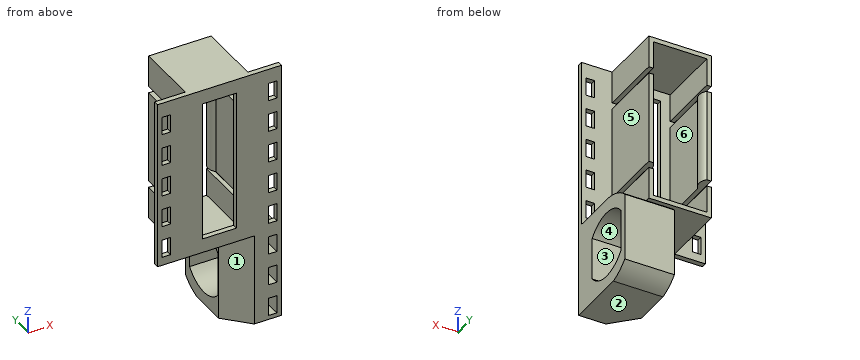
Autodesk Inventor part; units mm, degrees
ref_plane "YZ Plane" through (0, 0, 0) normal (1, 0, 0) x (0, 1, 0)
ref_plane "XZ Plane" through (0, 0, 0) normal (0, 1, 0) x (-1, 0, 0)
ref_plane "XY Plane" through (0, 0, 0) normal (0, 0, 1) x (1, 0, 0)
sketch "Sketch1" plane through (0, 0, 0) normal (0, 1, 0) x (-1, 0, 0)
  line L0 (-19.2, 26.4) -> (19.2, 26.4)
  line L1 (19.2, 26.4) -> (19.2, -26.4)
  line L2 (10.8, -26.4) -> (-10.8, -26.4)
  line L3 (-19.2, -26.4) -> (-19.2, 26.4)
  line L4 (-19.2, 26.4) -> (19.2, -26.4) construction
  line L5 (19.2, 26.4) -> (-19.2, -26.4) construction
  line L6 (-5.3, 22) -> (5.3, 22)
  line L7 (5.3, 22) -> (5.3, -22)
  line L8 (5.3, -22) -> (-5.3, -22)
  line L9 (-5.3, -22) -> (-5.3, 22)
  line L10 (-5.3, 22) -> (5.3, -22) construction
  line L11 (5.3, 22) -> (-5.3, -22) construction
  line L12 (-10.8, -26.4) -> (-10.8, -55.1)
  line L13 (-10.8, -55.1) -> (-19.2, -55.1)
  line L14 (-19.2, -55.1) -> (-19.2, -26.4)
  line L15 (10.8, -26.4) -> (19.2, -26.4)
  point P0 (0, 0)
  point P1 (13.2741, -55.1)
  dimension "d4" = 10.6
  dimension "d5" = 44
  dimension "d37" = 8.4
extrude "Extrusion1" add sketch "Sketch1" along normal blind 1.6
sketch "Sketch3" plane through (0, 1.6, 0) normal (0, 1, 0) x (1, 0, 0)
  line L0 (-5.3, 22) -> (5.3, 22)
  line L1 (5.3, -22) -> (-5.3, -22)
  line L2 (-19.2, -26.4) -> (19.2, -26.4)
  line L3 (10.8, 26.4) -> (-19.2, 26.4)
  line L4 (9.7, -26.4) -> (-9.7, -26.4)
  line L5 (-9.7, -26.4) -> (-9.7, 26.4)
  line L6 (-9.7, 26.4) -> (9.7, 26.4)
  line L7 (9.7, 26.4) -> (9.7, -26.4)
  line L8 (9.7, -26.4) -> (-9.7, 26.4) construction
  line L9 (-9.7, -26.4) -> (9.7, 26.4) construction
  line L10 (8.3, -25) -> (-8.3, -25)
  line L11 (-8.3, -25) -> (-8.3, 25)
  line L12 (-8.3, 25) -> (8.3, 25)
  line L13 (8.3, 25) -> (8.3, -25)
  line L14 (8.3, -25) -> (-8.3, 25) construction
  line L15 (-8.3, -25) -> (8.3, 25) construction
  line L16 (-9.7, 16.4) -> (-8.3, 16.4)
  line L17 (-9.7, 14.4) -> (-8.3, 14.4)
  line L18 (-9.7, -14.4) -> (-8.3, -14.4)
  line L19 (-9.7, -16.4) -> (-8.3, -16.4)
  line L20 (0, 22) -> (0, -22)
  line L21 (9.7, 16.4) -> (8.3, 16.4)
  line L22 (9.7, 14.4) -> (8.3, 14.4)
  line L23 (9.7, -14.4) -> (8.3, -14.4)
  line L24 (9.7, -16.4) -> (8.3, -16.4)
  line L25 (8.3, 16.4) -> (8.3, 14.4)
  line L26 (9.7, 16.4) -> (9.7, 14.4)
  line L27 (9.7, -14.4) -> (9.7, -16.4)
  line L28 (8.3, -14.4) -> (8.3, -16.4)
  point P0 (19.2, 26.4)
  point P1 (-10.8, 26.4)
  point P2 (0, 0)
  point P3 (0, 0)
  dimension "d8" = 19.4
  dimension "d9" = 1.4
  dimension "d10" = 1.4
  dimension "d11" = 2
  dimension "d12" = 10
  dimension "d13" = 2
  dimension "d14" = 10
extrude "Extrusion2" add sketch "Sketch3" along normal blind 20 contours L5 L19 L11 L10 L13 L24 L7 L2 | L5 L17 L11 L18 | L23 L13 L22 L7 | L5 L3 L7 L21 L13 L12 L11 L16
sketch "Sketch8" plane through (0, 1.6, 0) normal (0, 1, 0) x (1, 0, 0)
  line L0 (19.2, -26.4) -> (19.2, 55.1)
  line L1 (10.8, 55.1) -> (19.2, 55.1)
  line L2 (19.2, 55.1) -> (19.2, 26.4)
  line L3 (19.2, 26.4) -> (10.8, 26.4)
  line L4 (10.8, 26.4) -> (10.8, 55.1)
  point P0 (0, 0)
extrude "Extrusion6" add sketch "Sketch8" along normal blind 23.6
sketch "Sketch9" plane through (10.8, 0, -55.1) normal (-1, 0, 0) x (0, 0, 1)
  line L0 (28.7, 0) -> (0, 0)
  line L1 (28.7, 0) -> (28.7, 1.6)
  line L2 (28.7, 1.6) -> (28.7, 25.2)
  line L3 (0, 25.2) -> (28.7, 25.2)
  line L4 (0, 0) -> (0, 25.2)
  point P0 (55.1, 0)
extrude "Extrusion7" add sketch "Sketch9" along normal blind 7
sketch "Sketch10" plane through (19.2, 0, -55.1) normal (0, 0, -1) x (-1, 0, 0)
  line L0 (15.4, 0) -> (0, 0)
  line L1 (15.4, 25.2) -> (15.4, 0)
  line L2 (8.4, 0) -> (15.4, 7.2)
  point P0 (19.2, 0)
  dimension "d42" = 7.2
  dimension "d43" = 7
extrude "Extrusion8" cut sketch "Sketch10" against normal up to surface (28.7 mm away)
sketch "Sketch11" plane through (19.2, 0, 26.4) normal (1, 0, 0) x (0, 0, -1)
  line L0 (81.5, 0) -> (0, 0)
  line L1 (81.5, 0) -> (81.5, 25.2)
  line L2 (52.8, 25.2) -> (81.5, 25.2)
  line L3 (52.8, 1.6) -> (52.8, 25.2)
  line L4 (52.8, 7.4) -> (81.5, 7.4)
  line L5 (55.0793, 23) -> (79.6991, 23)
  arc A0 (60.8, 23) -> (60.8, 7.4) centre (67.0851, 15.2) ccw
  arc A1 (74, 7.4) -> (74, 23) centre (67.6284, 15.2) ccw
  arc A2 (56.8391, 25.2) -> (52.8, 16.1566) centre (67.0851, 15.2) ccw
  line L6 (52.8, 14.2434) -> (52.8, 7.4)
  line L7 (52.8, 7.4) -> (60.8, 7.4)
  line L8 (74.3931, 7.4) -> (81.5, 7.4)
  arc A3 (81.5, 18.9579) -> (77.9504, 25.2) centre (67.6284, 15.2) ccw
  line L9 (81.5, 11.4421) -> (81.5, 7.4)
  line L10 (77.9504, 25.2) -> (56.8391, 25.2)
  arc A4 (56.8391, 25.2) -> (52.8, 16.1566) centre (67.0851, 15.2) ccw
  line L11 (56.8391, 25.2) -> (52.8, 25.2)
  line L12 (52.8, 25.2) -> (52.8, 14.2434)
  line L13 (77.9504, 25.2) -> (81.5, 25.2)
  line L14 (81.5, 25.2) -> (81.5, 18.9579)
  arc A5 (56.8391, 25.2) -> (52.8, 16.1566) centre (67.0851, 15.2) ccw
  line L15 (52.8, 16.1566) -> (52.8, 25.2)
  line L16 (52.8, 25.2) -> (56.8391, 25.2)
  point P0 (26.4, 0)
  point P1 (77.7, 15.2)
  point P2 (57.1, 15.2)
  dimension "d46" = 7.4
  dimension "d47" = 2.2
  dimension "d48" = 8
  dimension "d49" = 13.2
  dimension "d50" = 7.8
  dimension "d51" = 3.7
  dimension "d52" = 8
  dimension "d53" = 13.2
  dimension "d54" = 7.8
  dimension "d55" = 3.7
  dimension "d56" = 4.3
  dimension "d57" = 4.3
extrude "Extrusion9" cut sketch "Sketch11" against normal up to surface (15.4 mm away) contours A3 L2 L1 | L4 A0 L5 A1 | A2 L3 L2
sketch "Sketch12" plane through (0, 0, 0) normal (0, -1, 0) x (1, 0, 0)
  line L0 (19.2, -55.1) -> (19.2, 26.4)
  line L1 (19.2, 26.4) -> (-19.2, 26.4)
  line L2 (-5.3, 22) -> (5.3, 22)
  line L3 (5.3, -22) -> (-5.3, -22)
  line L4 (15.2, 21.8) -> (17.8, 21.8)
  line L5 (17.8, 21.8) -> (17.8, 16.2)
  line L6 (17.8, 16.2) -> (15.2, 16.2)
  line L7 (15.2, 16.2) -> (15.2, 21.8)
  line L8 (0, 22) -> (0, -22)
  line L9 (15.2, 11.8) -> (17.8, 11.8)
  line L10 (17.8, 11.8) -> (17.8, 6.2)
  line L11 (17.8, 6.2) -> (15.2, 6.2)
  line L12 (15.2, 6.2) -> (15.2, 11.8)
  line L13 (15.2, 1.8) -> (17.8, 1.8)
  line L14 (17.8, 1.8) -> (17.8, -3.8)
  line L15 (17.8, -3.8) -> (15.2, -3.8)
  line L16 (15.2, -3.8) -> (15.2, 1.8)
  line L17 (15.2, -8.2) -> (17.8, -8.2)
  line L18 (17.8, -8.2) -> (17.8, -13.8)
  line L19 (17.8, -13.8) -> (15.2, -13.8)
  line L20 (15.2, -13.8) -> (15.2, -8.2)
  line L21 (15.2, -18.2) -> (17.8, -18.2)
  line L22 (17.8, -18.2) -> (17.8, -23.8)
  line L23 (17.8, -23.8) -> (15.2, -23.8)
  line L24 (15.2, -23.8) -> (15.2, -18.2)
  line L25 (15.2, -28.2) -> (17.8, -28.2)
  line L26 (17.8, -28.2) -> (17.8, -33.8)
  line L27 (17.8, -33.8) -> (15.2, -33.8)
  line L28 (15.2, -33.8) -> (15.2, -28.2)
  line L29 (15.2, -38.2) -> (17.8, -38.2)
  line L30 (17.8, -38.2) -> (17.8, -43.8)
  line L31 (17.8, -43.8) -> (15.2, -43.8)
  line L32 (15.2, -43.8) -> (15.2, -38.2)
  line L33 (15.2, -48.2) -> (17.8, -48.2)
  line L34 (17.8, -48.2) -> (17.8, -53.8)
  line L35 (17.8, -53.8) -> (15.2, -53.8)
  line L36 (15.2, -53.8) -> (15.2, -48.2)
  line L37 (-15.2, 21.8) -> (-17.8, 21.8)
  line L38 (-17.8, 21.8) -> (-17.8, 16.2)
  line L39 (-17.8, 16.2) -> (-15.2, 16.2)
  line L40 (-15.2, 16.2) -> (-15.2, 21.8)
  line L41 (-15.2, 11.8) -> (-17.8, 11.8)
  line L42 (-17.8, 11.8) -> (-17.8, 6.2)
  line L43 (-15.2, 6.2) -> (-15.2, 11.8)
  line L44 (-17.8, 6.2) -> (-15.2, 6.2)
  line L45 (-15.2, 1.8) -> (-17.8, 1.8)
  line L46 (-17.8, 1.8) -> (-17.8, -3.8)
  line L47 (-15.2, -3.8) -> (-15.2, 1.8)
  line L48 (-17.8, -3.8) -> (-15.2, -3.8)
  line L49 (-15.2, -8.2) -> (-17.8, -8.2)
  line L50 (-17.8, -8.2) -> (-17.8, -13.8)
  line L51 (-15.2, -13.8) -> (-15.2, -8.2)
  line L52 (-17.8, -13.8) -> (-15.2, -13.8)
  line L53 (-15.2, -18.2) -> (-17.8, -18.2)
  line L54 (-17.8, -18.2) -> (-17.8, -23.8)
  line L55 (-15.2, -23.8) -> (-15.2, -18.2)
  line L56 (-17.8, -23.8) -> (-15.2, -23.8)
  point P0 (0, 0)
  dimension "d60" = 1.4
  dimension "d61" = 5.6
  dimension "d62" = 4.6
  dimension "d63" = 2.6
  dimension "d66" = 10
extrude "Extrusion10" cut sketch "Sketch12" against normal blind 5
sketch "Sketch13" plane through (8.3, 1.6, -14.4) normal (-1, 0, 0) x (0, 0, 1)
  line L0 (28.8, 0) -> (28.8, 20)
  line L1 (0, 20) -> (28.8, 20)
  line L2 (0, 20) -> (28.8, 20)
  line L3 (28.8, 20) -> (28.8, 15)
  line L4 (28.8, 15) -> (0, 15)
  line L5 (0, 15) -> (0, 20)
  point P0 (14.4, -1.6)
  dimension "d73" = 5
extrude "Extrusion11" add sketch "Sketch13" along normal blind 5
sketch "Sketch14" plane through (8.3, 1.6, 14.4) normal (0, 0, 1) x (1, 0, 0)
  line L0 (1.4, 20) -> (-5, 20)
  line L1 (-5, 15) -> (-5, 20)
  line L2 (0, 15) -> (-5, 15)
  line L3 (0, 15) -> (0, 20)
  arc A0 (0, 20) -> (0, 15) centre (2.625, 17.5) ccw
  point P0 (-8.3, -1.6)
  point P1 (-1, 17.5)
  dimension "d76" = 1
extrude "Extrusion12" cut sketch "Sketch14" against normal up to surface (28.8 mm away) contours A0 L2 L1 L0
mirror "Mirror1" about plane through (0, 0, 0) normal (1, 0, 0) of "Extrusion11", "Extrusion12"
properties part number "motor housing"
Verification items for the finished model (mm, model axes). Face numbers are marked on the shaded views. A direction names the side the tool comes from. Coordinates: 2 decimals unless noted, no trailing zeros. Order: outer loops, then holes, each group sorted by start corner. A loop starts at its lowest first (then second) coordinate and runs counter-clockwise, first axis right, second up. Notation, with made-up numbers: (9, 15.25) -> (18, 15.25) arc R29 ccw to (18, 44.25) -> close; hole circle Ø10 at (65.5, 34). An arc over 180 degrees is marked (long way). Put each result on its own line as item: value. Start each with the question number.
1. Cross-section at A-A, the plane x = -3. Record the boundary of the cut face in (y, z), then the cut area to 3 significant figures.
2. Cross-section at C-C, the plane z = -36.5. Record the boundary of the cut face in (x, y), then the cut area to 3 significant figures.
3. Material ranges on L1, parallel to Z at x = -9, y = 2.75; L2, parallel to Y at x = 15, z = -38.5; L3, parallel to X at y = 10.75, z = -19.5, recorded low to high. Write a range as [from, to].
4. Mould release check, pull along Y, two halves, no side actions. Record for the marked faces 1, 2 and 3: released by +Y, released by -Y, zero draft, split by the parting line, or undercut.
5. Cross-section at D-D, the plane y = 11.5. Count the separate pieces of the cut face and the enclosed holes in it, then the cut area to 3 significant figures.
6. Go/stop test with flat-tipped pins: pin 1 Ø5 at (y, z) = (22, 12.5) entering from -X; pin 2 Ø5.5 at (y, z) = (3.5, -41.5) entering from -X; pin 3 Ø5 at (x, z) = (2, 5.5) entering from +Y; pin 4 Ø3 at (x, y) = (15.5, 6) entering from +Z. Record where each tip stops, or that it passes through.
7. Cross-section at B-B, the plane z = 20. Record the boundary of the cut face in (x, y).
8. Access from +Z, -Z, +X, -X, +Y, -Y to the whole of each face (thin tool, end or side, straight path). Record for the marked faces 4, 5 and 6.
Computed:
1. outline: (0, -26.4) -> (21.6, -26.4) -> (21.6, -25) -> (1.6, -25) -> (1.6, -22) -> (0, -22) -> close; (0, 22) -> (1.6, 22) -> (1.6, 25) -> (21.6, 25) -> (21.6, 26.4) -> (0, 26.4) -> close
1. area: 70.1 mm2
2. outline: (3.8, 7.2) -> (10.8, 0) -> (19.2, 0) -> (19.2, 7.4) -> (3.8, 7.4) -> close; (3.8, 23) -> (19.2, 23) -> (19.2, 25.2) -> (3.8, 25.2) -> close
2. area: 123 mm2
3. L1: [-26.4, -16.4], [-14.4, 14.4], [16.4, 26.4]
3. L2: [0, 7.4], [23, 25.2]
3. L3: [-9.7, -8.3], [8.3, 9.7]
4. face 1: released by -Y
4. face 2: zero draft
4. face 3: undercut
5. separate pieces: 5
5. enclosed holes: 0
5. area: 329 mm2
6. pin 1: x = -9.7
6. pin 2: x = 4.72
6. pin 3: through
6. pin 4: z = -26.4
7. outline: (-19.2, 0) -> (-17.8, 0) -> (-17.8, 1.6) -> (-19.2, 1.6) -> close; (-15.2, 0) -> (-5.3, 0) -> (-5.3, 1.6) -> (-8.3, 1.6) -> (-8.3, 21.6) -> (-9.7, 21.6) -> (-9.7, 1.6) -> (-15.2, 1.6) -> close; (5.3, 0) -> (15.2, 0) -> (15.2, 1.6) -> (9.7, 1.6) -> (9.7, 21.6) -> (8.3, 21.6) -> (8.3, 1.6) -> (5.3, 1.6) -> close; (17.8, 0) -> (19.2, 0) -> (19.2, 1.6) -> (17.8, 1.6) -> close
8. face 4: +X, -X
8. face 5: +Z, +X, +Y
8. face 6: none
